Geometry: final body of the model. Coordinates: model frame, mm. A direction names the side the tool comes from. Give positions to 0.01 mm unless a question says otherwise; leave off trailing zeros. Loops run counter-clockwise (first coordinate to the right, second up) from the corner with the lowest first, then second, coordinate; pieces in that order, holes last. Notation, with made-up numbers: M 62.25,30.25 L 89.25,30.25 A14 cw 89.25,43.25 Z; hole C 17.5,5.25 d11. An arc over 180 degrees is marked long. Put each result on its own line as item: value.
```python
from build123d import *

# Parameters (mm, degrees)
BOSS_EXTRUDE1_DEPTH            = 0.75
FILLET1_R                      = 2
F_3_2_3_2_DIAMETER_HOLE1_D     = 3.2
F_3_2_3_2_DIAMETER_HOLE1_DEPTH = 10
F_3_2_3_2_DIAMETER_HOLE1_TIP   = 0.96137699
CUT_EXTRUDE1_DEPTH             = 1.5
FILLET2_R                      = 2


with BuildPart() as part:
    # Sketch1 → Boss-Extrude1 (new body, symmetric)
    with BuildSketch(Plane(origin=(0, 0, 0), x_dir=(1, 0, 0), z_dir=(0, 1, 0))):
        with BuildLine():
            Line((-18.5, -22), (18.5, -22))
            ThreePointArc((18.5, -22), (24.474873734, -24.474873734), (22, -18.5))
            Line((22, -18.5), (22, 18.5))
            ThreePointArc((22, 18.5), (24.474873734, 24.474873734), (18.5, 22))
            Line((18.5, 22), (-18.5, 22))
            ThreePointArc((-18.5, 22), (-24.474873734, 24.474873734), (-22, 18.5))
            Line((-22, 18.5), (-22, -18.5))
            ThreePointArc((-22, -18.5), (-24.474873734, -24.474873734), (-18.5, -22))
        make_face()
    extrude(amount=BOSS_EXTRUDE1_DEPTH, both=True)

    # Fillet1
    fillet1_edges = [part.edges().sort_by_distance(p)[0] for p in [
        (-18.5, 0, -22),
        (18.5, 0, -22),
        (22, 0, -18.5),
        (22, 0, 18.5),
        (18.5, 0, 22),
        (-18.5, 0, 22),
        (-22, 0, 18.5),
        (-22, 0, -18.5),
    ]]
    fillet(fillet1_edges, radius=FILLET1_R)

    # Ø3.2 (3.2) Diameter Hole1
    with Locations(Plane(origin=(0, 0.75, 0), x_dir=(1, 0, 0), z_dir=(0, 1, 0))):
        with Locations((-22, 22), (-22, -22), (22, -22), (22, 22)):
            Hole(F_3_2_3_2_DIAMETER_HOLE1_D / 2, depth=F_3_2_3_2_DIAMETER_HOLE1_DEPTH)
            with Locations((0, 0, -(F_3_2_3_2_DIAMETER_HOLE1_DEPTH + F_3_2_3_2_DIAMETER_HOLE1_TIP / 2))):  # 118° drill point
                Cone(0, F_3_2_3_2_DIAMETER_HOLE1_D / 2, F_3_2_3_2_DIAMETER_HOLE1_TIP, mode=Mode.SUBTRACT)

    # Sketch4 → Cut-Extrude1 (cut)
    with BuildSketch(Plane(origin=(0, 0.75, 0), x_dir=(1, 0, 0), z_dir=(0, 1, 0))):
        Polygon((-1.414213562, 0), (-15, 13.585786438), (-15, -13.585786438), align=None)
        Polygon((13.585786438, 15), (-13.585786438, 15), (0, 1.414213562), align=None)
        Polygon((15, -13.585786438), (15, 13.585786438), (1.414213562, 0), align=None)
        Polygon((0, -1.414213562), (-13.585786438, -15), (13.585786438, -15), align=None)
    extrude(amount=-CUT_EXTRUDE1_DEPTH, mode=Mode.SUBTRACT)

    # Fillet2
    fillet2_edges = [part.edges().sort_by_distance(p)[0] for p in [
        (-1.414213562, 0, 0),
        (-15, 0, 13.585786438),
        (-15, 0, -13.585786438),
        (13.585786438, 0, -15),
        (0, 0, -1.414213562),
        (-13.585786438, 0, -15),
        (15, 0, -13.585786438),
        (15, 0, 13.585786438),
        (1.414213562, 0, 0),
        (0, 0, 1.414213562),
        (13.585786438, 0, 15),
        (-13.585786438, 0, 15),
    ]]
    fillet(fillet2_edges, radius=FILLET2_R)


solid = part.part
```
Item 1: Section D-D on z = -21. Output: boundary loops of the cut face in (x, y).
Output values:
outline: M -25.35,-0.75 L -23.25,-0.75 L -23.25,0.75 L -25.35,0.75 Z; M -20.75,-0.75 L 20.75,-0.75 L 20.75,0.75 L -20.75,0.75 Z; M 23.25,-0.75 L 25.35,-0.75 L 25.35,0.75 L 23.25,0.75 Z
Item 2: Set-up query: faces 1 (the flat face through (0, 0, -22)), 2 (the flat face through (22, 0, 0)), 3 (the cylindrical face through (-10.62, -0.01, 13.73)), 4 (the cylindrical face through (-17.99, -0.01, 22.34)), 5 (the flat face through (-22, 0, 0)). Return all of +Z, -Z, +X, -X, +Y, -Y with unobstructed straight access to the full face (end or side cutting, diameter ignored); none if empty.
Output values:
face 1: -Z, +Y, -Y
face 2: +X, +Y, -Y
face 3: +Y, -Y
face 4: +Z, +Y, -Y
face 5: -X, +Y, -Y
Item 3: Section B-B on z = 8. Output: boundary loops of the cut face in (x, y), then the cut area to 3 significant figures.
Output values:
outline: M -22,-0.75 L -15,-0.75 L -15,0.75 L -22,0.75 Z; M -9.41,-0.75 L -6.59,-0.75 L -6.59,0.75 L -9.41,0.75 Z; M 6.59,-0.75 L 9.41,-0.75 L 9.41,0.75 L 6.59,0.75 Z; M 15,-0.75 L 22,-0.75 L 22,0.75 L 15,0.75 Z
area: 29.5 mm²
Item 4: Mould query, pull axis Z, two halves, no side actions, for faces 6 (the cylindrical face through (17.99, 0.01, -22.34)), 7 (the flat face through (-7.268, 0.01, 5.854)), 8 (the flat face through (0, 0, 22)). Classes: pulls with the +Z half, pulls with the -Z half, needs draft (parallel to the pull), parting line crosses it, or undercut.
Output values:
face 6: pulls with the -Z half
face 7: undercut
face 8: pulls with the +Z half
Item 5: Pin query (flat end, axial travel): pin 1 Ø0.8 at (x, y) = (2, -0.5) entering from -Z; pin 2 Ø3.5 at (x, z) = (22, -22) entering from -Y. Return the tip coordinate at first contact, or that it passes through.
Output values:
pin 1: z = -22
pin 2: y = -0.75
Item 6: Section C-C on y = 0.35. Count the separate pieces of the cut face and the enclosed holes in it, then the cut area to 3 significant figures.
Output values:
separate pieces: 1
enclosed holes: 8
area: 1,330 mm²
Item 7: Line query: probe 1 along X at (y, z) = (0.4, -21); probe 2 along X at (y, z) = (0, 10). Output: solid intervals per line, ascending. Write a range as [from, to].
Output values:
probe 1: [-25.35, -23.25], [-20.75, 20.75], [23.25, 25.35]
probe 2: [-22, -14.57], [-11.41, -8.59], [8.59, 11.41], [14.57, 22]
Item 8: Section A-A on x = -8. Output: boundary loops of the cut face in (y, z), then the cut area to 3 significant figures.
Output values:
outline: M -0.75,-22 L 0.75,-22 L 0.75,-15 L -0.75,-15 Z; M -0.75,-9.41 L 0.75,-9.41 L 0.75,-6.59 L -0.75,-6.59 Z; M -0.75,6.59 L 0.75,6.59 L 0.75,9.41 L -0.75,9.41 Z; M -0.75,15 L 0.75,15 L 0.75,22 L -0.75,22 Z
area: 29.5 mm²
